Verification items for this drawing (mm, ordinates from the low corner). Give positions to 0.01 mm unless a question says otherwise; leave off trailing zeros. Write each loop counter-clockwise with the first axis right and the second up, starting at its lowest first coordinate (ties: lowest second). Pieces come first, ordered by that corner, then holes. Notation, with made-up numbers: M 66.25,81 L 94.25,81 A12 cw 94.25,103 Z; hole C 79,89 d11. An arc over 180 degrees is marked long. Write each question's results on one line, items separated by ' | '.
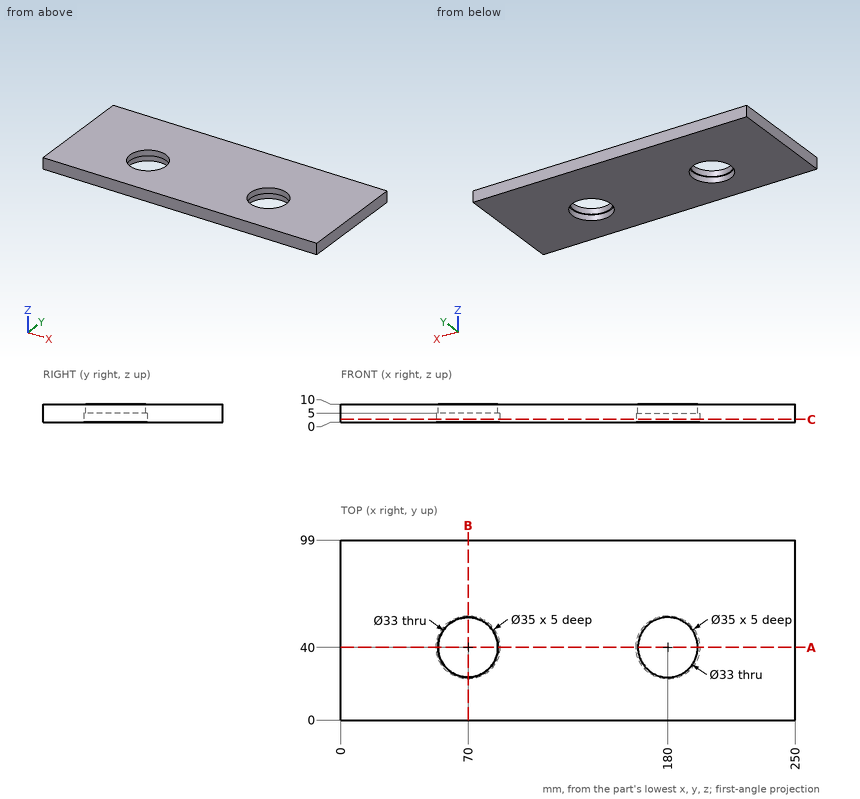
Q1. Section check C-C (z = 1.5). Enter the section's corners in (x, y), then the cut area to 3 significant figures.
Answer key:
outline: M 0,0 L 250,0 L 250,99 L 0,99 Z; hole C 70,40 d35; hole C 180,40 d35 | area: 22,800 mm2
Q2. Material ranges on probe 1 along Y at (x, z) = (180, 7.6); probe 2 along Y at (x, z) = (180, 3.7); probe 3 along X at (y, z) = (28, 2.5), recorded low to high. Write a range as [from, to].
Answer key:
probe 1: y = [0, 23.5], [56.5, 99] | probe 2: y = [0, 22.5], [57.5, 99] | probe 3: x = [0, 57.26], [82.74, 167.26], [192.74, 250]
Q3. Section check B-B (x = 70). Enter the section's corners in (y, z), then the cut area to 3 significant figures.
Answer key:
outline: M 0,0 L 22.5,0 L 22.5,5 L 23.5,5 L 23.5,10 L 0,10 Z; M 56.5,5 L 57.5,5 L 57.5,0 L 99,0 L 99,10 L 56.5,10 Z | area: 650 mm2
Q4. Section check A-A (y = 40). Enter the section's corners in (x, z).
Answer key:
outline: M 0,0 L 52.5,0 L 52.5,5 L 53.5,5 L 53.5,10 L 0,10 Z; M 86.5,5 L 87.5,5 L 87.5,0 L 162.5,0 L 162.5,5 L 163.5,5 L 163.5,10 L 86.5,10 Z; M 196.5,5 L 197.5,5 L 197.5,0 L 250,0 L 250,10 L 196.5,10 Z
